from build123d import *

# Parameters (mm, degrees)
SKETCH070_W             = 70
SKETCH070_H             = 100
PAD024_DEPTH            = 10
SKETCH071_R             = 1.5
POCKET046_DEPTH         = 70.001
CHAMFER006_SIZE         = 1
BODY020_PLACEMENT_ANGLE = 180


with BuildPart() as part:
    # Sketch070 → Pad024 (new body)
    with BuildSketch(Plane.XY):
        Rectangle(SKETCH070_W, SKETCH070_H)
    extrude(amount=PAD024_DEPTH)

    # Sketch071 (on Face3 of Pad024) → Pocket046 (cut, through all)
    with BuildSketch(Plane.YZ.offset(35)):
        with Locations((36, 3)):
            Circle(SKETCH071_R)
        with Locations((-41, 3)):
            Circle(SKETCH071_R)
    extrude(amount=-POCKET046_DEPTH, mode=Mode.SUBTRACT)

    # Chamfer006
    chamfer006_edges = [part.edges().sort_by_distance(p)[0] for p in [
        (-35, 0, 0),
        (0, -50, 0),
        (35, 0, 0),
        (0, 50, 0),
        (-35, 0, 10),
        (0, -50, 10),
        (35, 0, 10),
        (0, 50, 10),
    ]]
    chamfer(chamfer006_edges, length=CHAMFER006_SIZE)


with BuildPart() as part_1:
    # Body020 placement: moved
    add(part.part.moved(Location((63.5, 55.3, 56.5))).rotate(Axis((63.5, 55.3, 56.5), (0, 0, 1)), BODY020_PLACEMENT_ANGLE))


solid = part_1.part
Design review of the part built by this model. Coordinates are the model's own, in mm. Coordinates: 2 decimals unless noted, no trailing zeros. Loops run counter-clockwise (first coordinate to the right, second up) from the corner with the lowest first, then second, coordinate; pieces in that order, holes last. Notation, with made-up numbers: (70, 57) -> (112, 57) arc R22 ccw to (112, 73) -> close; hole circle Ø7 at (83.25, 63.25). An arc over 180 degrees is marked (long way). Use a Markdown table: item, result. Add a question column.
Item 1: The part is to be moulded in two halves that separate along Y. For faces 1 (the flat face through (64, 5.3, 61)), 2 (the cylindrical face through (63.01, 97.41, 60.51)), 3 (the flat face through (64, 105.3, 61)), say which applies: +Y half, -Y half, draft (parallel to the pull), parting line (faces both ways), or undercut.
Item 2: Clearance check with a flat-ended pin moving along its axis: P1, Ø2.5, axis at y = 96.3, z = 59.5, coming from the -X side. State where the tip first meets the part, or that it passes through.
Item 3: We need section A-A, the plane z = 59.5. Write out the cut boundary in (x, y).
Item 4: We need section C-C, the plane x = 84. Write out the cut boundary in (y, z), and give its area (3 significant figures).
Item 5: We need section B-B, the plane y = 96.3. Write out the cut boundary in (x, z), and give its area (3 significant figures).
Item 6: Wall thickness on L1, parallel to Z at x = 56, y = 96.3; L2, parallel to X at y = 99, z = 57: over which ranges is each line inside the solid? List them lowest first. Write a range as from..to.
Numbers:
| question | item | result |
|---|---|---|
| 1 | face 1 | -Y half |
| 1 | face 2 | undercut |
| 1 | face 3 | +Y half |
| 2 | P1 | passes through |
| 3 | outline | (28.5, 5.3) -> (98.5, 5.3) -> (98.5, 17.8) -> (28.5, 17.8) -> close; (28.5, 20.8) -> (98.5, 20.8) -> (98.5, 94.8) -> (28.5, 94.8) -> close; (28.5, 97.8) -> (98.5, 97.8) -> (98.5, 105.3) -> (28.5, 105.3) -> close |
| 4 | outline | (5.3, 57.5) -> (6.3, 56.5) -> (104.3, 56.5) -> (105.3, 57.5) -> (105.3, 65.5) -> (104.3, 66.5) -> (6.3, 66.5) -> (5.3, 65.5) -> close; hole circle Ø3 at (19.3, 59.5); hole circle Ø3 at (96.3, 59.5) |
| 4 | area | 984 mm^2 |
| 5 | outline | (28.5, 57.5) -> (29.5, 56.5) -> (97.5, 56.5) -> (98.5, 57.5) -> (98.5, 58) -> (28.5, 58) -> close; (28.5, 61) -> (98.5, 61) -> (98.5, 65.5) -> (97.5, 66.5) -> (29.5, 66.5) -> (28.5, 65.5) -> close |
| 5 | area | 488 mm^2 |
| 6 | L1 | z = 56.5..58, 61..66.5 |
| 6 | L2 | x = 29..98 |
